from build123d import *

# Parameters (mm, degrees)
SKETCH058_R             = 12.2936
PAD026_DEPTH            = 47.752
PAD027_DEPTH            = 25.2222
SKETCH062_R             = 3.4925
PAD029_DEPTH            = 2.54
BODY021_PLACEMENT_ANGLE = 180


with BuildPart() as part:
    # Sketch058 → Pad026 (new body)
    with BuildSketch(Plane.YZ):
        Circle(SKETCH058_R)
    extrude(amount=PAD026_DEPTH)

    # Sketch059 (on Face2 of Pad026) → Pad027 (join)
    with BuildSketch(Plane(origin=(0, 0, 0), x_dir=(0, 1, 0), z_dir=(-1, 0, 0))):
        with BuildLine():
            ThreePointArc((-1.524, 1.078304), (0, -1.8669), (1.524, 1.078304))
            Line((-1.524, 1.078304), (1.524, 1.078304))
        make_face()
    extrude(amount=PAD027_DEPTH)

    # Sketch062 (on Face2 of Pad027) → Pad029 (join)
    with BuildSketch(Plane(origin=(0, 0, 0), x_dir=(0, 1, 0), z_dir=(-1, 0, 0))):
        Circle(SKETCH062_R)
    extrude(amount=PAD029_DEPTH)


with BuildPart() as part_1:
    # Body021 placement: moved
    add(part.part.moved(Location((-0.1778, 40.259, 0.5588))).rotate(Axis((-0.1778, 40.259, 0.5588), (0, 0, 1)), BODY021_PLACEMENT_ANGLE))


solid = part_1.part
CAD build for the part. Positions are in the model's coordinates, mm. A direction names the side the tool comes from. Give positions to 0.01 mm unless a question says otherwise; leave off trailing zeros. Order: outer loops, then holes, each group sorted by start corner. A loop starts at its lowest first (then second) coordinate and runs counter-clockwise, first axis right, second up. Notation, with made-up numbers: (-33.75, 52) - (-22.75, 52) arc R32 cw to (-22.75, 89) - close; hole circle Ø10 at (1, -34). An arc over 180 degrees is marked (long way). Answer in a Markdown table with one row per item.
1. Pull direction Z, two halves, no side cores. Call faces 3 (the cylindrical face through (1.07, 43.75, 0.41)), 4 (the flat face through (25.044, 40, 1)), 5 (the flat face through (14, 40, -0.52)): pulls with the +Z half, pulls with the -Z half, needs draft (parallel to the pull), parting line crosses it, or undercut.
Data:
| item | result |
|---|---|
| face 3 | parting line crosses it |
| face 4 | needs draft |
| face 5 | pulls with the -Z half |
2. Tool access for faces 1 (the cylindrical face through (13.545, 40.316, 2.425)), 2 (the flat face through (-47.93, 40, 1)): list every direction of +Z, -Z, +X, -X, +Y, -Y with a clear straight run to the whole face (end or side of a thin tool).
Data:
| item | result |
|---|---|
| face 1 | +X |
| face 2 | +Z, -Z, -X, +Y, -Y |
3. Saw through at D-D, the plane y = 37.5. Give the cut face in (x, z).
Data:
| item | result |
|---|---|
| outline | (-47.93, -11.42) - (-0.18, -11.42) - (-0.18, -1.58) - (2.36, -1.58) - (2.36, 2.7) - (-0.18, 2.7) - (-0.18, 12.54) - (-47.93, 12.54) - close |
4. Saw through at B-B, the plane x = 20. Give the cut face in (y, z) (1 decimal), plus the area to 3 significant figures.
Data:
| item | result |
|---|---|
| outline | (38.7, -0.5) - (41.8, -0.5) arc R1.9 ccw (long way) to start |
| area | 9.26 mm² |
5. Saw through at C-C, the plane z = 8.5. Give the cut face in (x, y), plus the area to 3 significant figures.
Data:
| item | result |
|---|---|
| outline | (-47.93, 30.87) - (-0.18, 30.87) - (-0.18, 49.64) - (-47.93, 49.64) - close |
| area | 896 mm² |
6. Saw through at A-A, the plane y = 40.75. Give the cut face in (x, z) (1 decimal), plus the area to 3 significant figures.
Data:
| item | result |
|---|---|
| outline | (-47.9, -11.7) - (-0.2, -11.7) - (-0.2, -2.9) - (2.4, -2.9) - (2.4, -0.5) - (25, -0.5) - (25, 2.4) - (2.4, 2.4) - (2.4, 4) - (-0.2, 4) - (-0.2, 12.8) - (-47.9, 12.8) - close |
| area | 1,260 mm² |
7. Probe probe 1 along X at (y, z) = (45, 7.5); probe 2 along Z at (x, y) = (-43.5, 40.25); probe 3 along X at (y, z) = (42.5, 2.25). List the from-to ranges inside material, lowest first. Write a range as [from, to].
Data:
| item | result |
|---|---|
| probe 1 | x = [-47.93, -0.18] |
| probe 2 | z = [-11.73, 12.85] |
| probe 3 | x = [-47.93, 2.36] |
8. Flat gauge pins, fed straight in: pin 1 (4 mm diameter, centred on x = -18.5, y = 48, fed in from +Z); pin 2 (12 mm diameter, centred on x = -7.5, y = 31, fed in from -Z); pin 3 (5 mm diameter, centred on x = -24, z = 5.5, fed in from -Y). Where does each tip first touch, or does it go through?
Data:
| item | result |
|---|---|
| pin 1 | stops at z = 11.43 |
| pin 2 | stops at z = -11.29 |
| pin 3 | stops at y = 28.21 |
